Input: dimensioned drawing with shaded views. Units: mm. Origin: part minimum x, y, z. A direction names the side the tool comes from. Round coordinates to 2 decimals unless told otherwise and drop trailing zeros. Write each loop counter-clockwise with the first axis right and the second up, starting at its lowest first coordinate (ties: lowest second). Pieces come first, ordered by that corner, then holes. Notation, with made-up numbers: (60.5, 52) -> (66.5, 52) arc R36 ccw to (66.5, 87) -> close; hole circle Ø4 at (26, 64). An arc over 180 degrees is marked (long way). Use one line per item in the form item = value. Start each with the question number.
1. Line query: L1, parallel to X at y = 394, z = 74.5; L2, parallel to Z at x = 264.5, y = 569 (1 decimal); L3, parallel to Y at x = 371, z = 164 (1 decimal). Output: solid intervals per line, ascending.
2. Reachability of the marked faces 1, 2 and 3 from +Z, -Z, +X, -X, +Y, -Y: full face, straight path, thin tool, end or side. Return the list, or none.
3. Cut plane D-D, the plane z = 259. Return the cut outline in (x, y).
4. Cut plane A-A, the plane z = 146. Return the cut outline in (x, y) (1 decimal).
5. Pin query (flat end, axial travel): pin 1 Ø4 at (y, z) = (140, 171.5) entering from +X. Return the tip coordinate at first contact, or that it passes through.
6. Cut plane C-C, the plane y = 98.5. Return the cut outline in (x, z), plus the area to 3 significant figures.
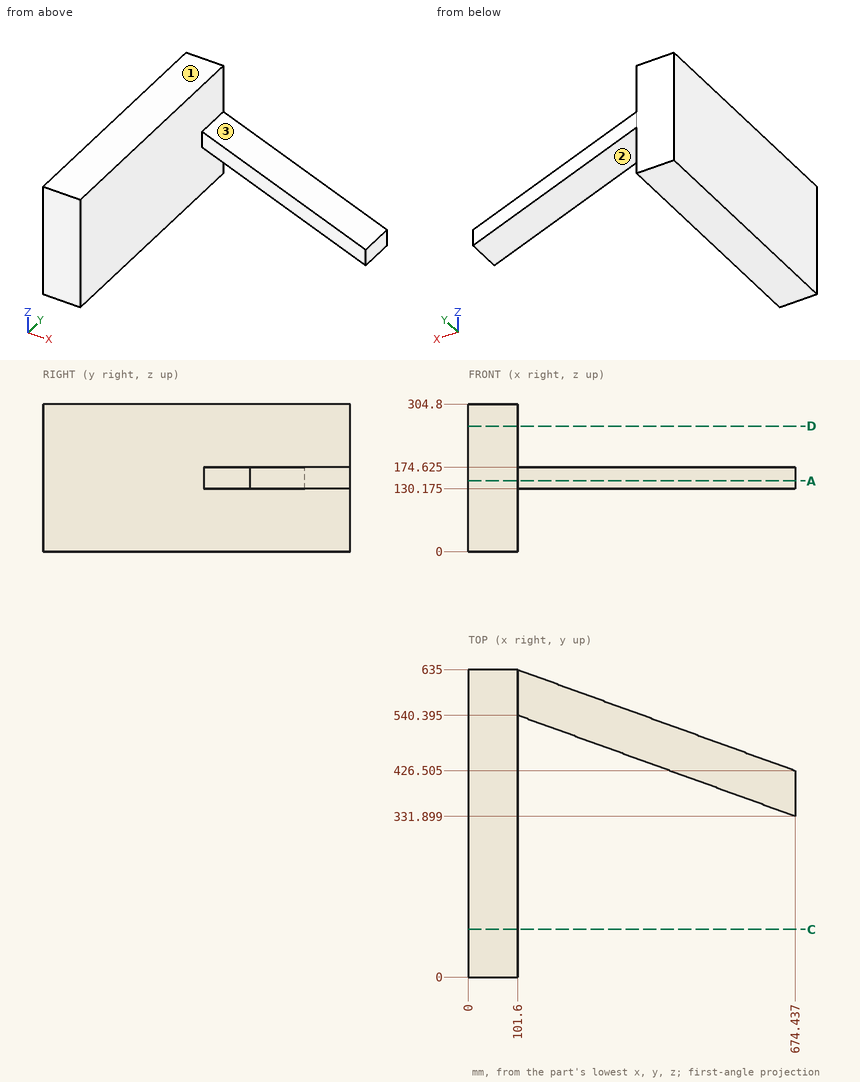
Outcome:
q1.L1 = 0 to 101.6
q1.L2 = 130.2 to 174.6
q1.L3 = 442.3 to 536.9
q2.face_1 = +Z, +X, -X, +Y, -Y
q2.face_2 = -Z, +X, +Y, -Y
q2.face_3 = +Z, +X, +Y, -Y
q3.outline = (0, 0) -> (101.6, 0) -> (101.6, 635) -> (0, 635) -> close
q4.outline = (0, 0) -> (101.6, 0) -> (101.6, 540.4) -> (674.4, 331.9) -> (674.4, 426.5) -> (101.6, 635) -> (0, 635) -> close
q5.pin_1 = 101.6
q6.outline = (0, 0) -> (101.6, 0) -> (101.6, 304.8) -> (0, 304.8) -> close
q6.area = 31,000 mm^2
